Drawing for the job (mm, zero at the part's lowest x, y, z). Give positions to 0.01 mm unless a question says otherwise; leave off trailing zeros. Order: outer loops, then holes, each group sorted by start corner. A loop starts at its lowest first (then second) coordinate and runs counter-clockwise, first axis right, second up. Notation, with made-up numbers: (0, 84.5) - (9, 84.5) arc R18 ccw to (9, 115.5) - close; hole circle Ø10 at (49, 27). An arc over 180 degrees is marked (long way). One line per item, written item: value.
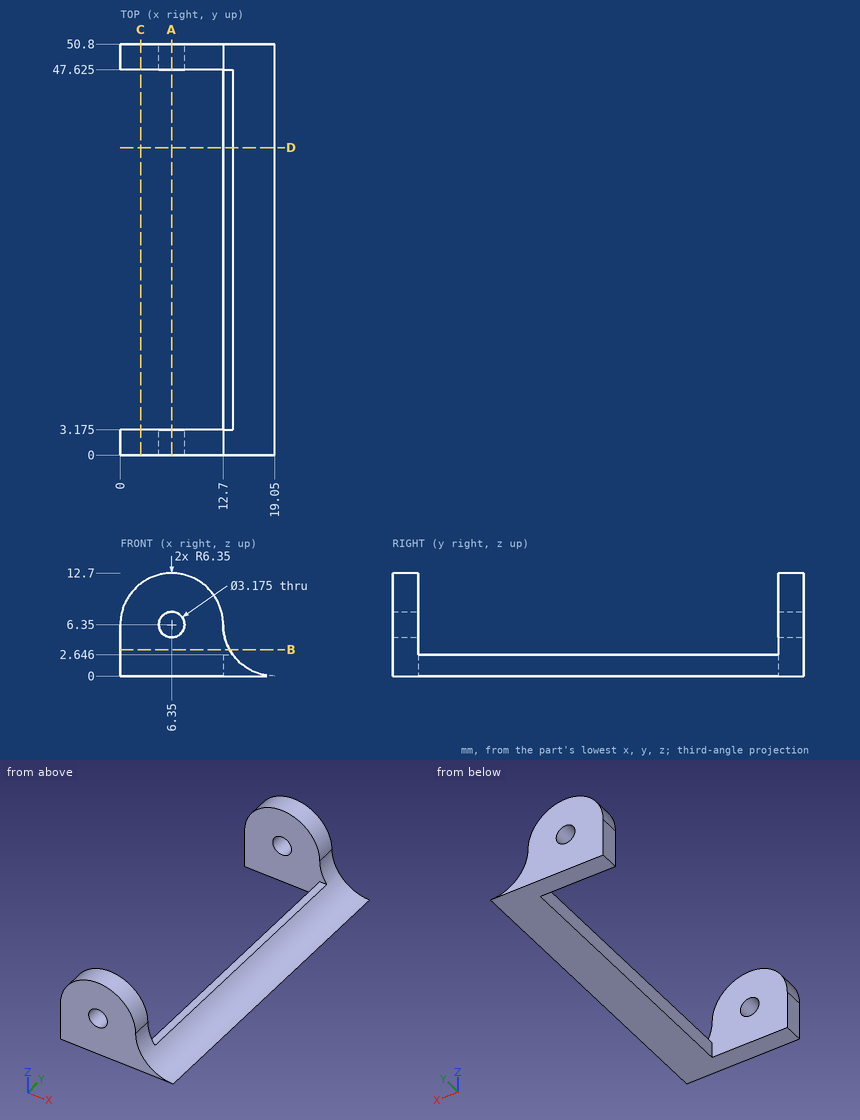
1) Cut at A-A, the plane x = 6.35. Give the cut face in (y, z) (1 decimal).
Outcome:
outline: (0, 0) - (3.2, 0) - (3.2, 4.8) - (0, 4.8) - close; (0, 7.9) - (3.2, 7.9) - (3.2, 12.7) - (0, 12.7) - close; (47.6, 0) - (50.8, 0) - (50.8, 4.8) - (47.6, 4.8) - close; (47.6, 7.9) - (50.8, 7.9) - (50.8, 12.7) - (47.6, 12.7) - close
2) Cut at C-C, the plane x = 2.5. Give the cut face in (y, z) (1 decimal).
Outcome:
outline: (0, 0) - (3.2, 0) - (3.2, 11.4) - (0, 11.4) - close; (47.6, 0) - (50.8, 0) - (50.8, 11.4) - (47.6, 11.4) - close
3) Drill centre lines: line 1 along Z through (x, y) = (6.35, 1.65); line 2 along Y through (x, z) = (10.75, 4.75) (3 decimals); line 3 along X through (y, z) = (48, 6.5). Where is each one in solid material? Low to high. Write a range as from..to.
Outcome:
line 1: z = 0..4.76, 7.94..12.7
line 2: y = 0..3.175, 47.625..50.8
line 3: x = 0..4.77, 7.93..12.7
4) Cut at D-D, the plane y = 38. Give the cut face in (x, z).
Outcome:
outline: (12.7, 0) - (19.05, 0) arc R6.35 cw to (13.89, 2.65) - (12.7, 2.65) - close
5) Pin check, flat tips, straight feed: pin 1 (1.5 mm diameter, centred on x = 10.5, y = 41.5, fed in from -Z); pin 2 (1 mm diameter, centred on x = 13.5, y = 17, fed in from +Z); pin 3 (2 mm diameter, centred on y = 18.5, z = 1.5, fed in from -X). Stop position of each tip, or through.
Outcome:
pin 1: passes through
pin 2: stops at z = 2.65
pin 3: stops at x = 12.7
6) Cut at B-B, the plane z = 3.25. Give the cut face in (x, y) (3 decimals), then the cut area to 3 significant figures.
Outcome:
outline: (0, 0) - (13.508, 0) - (13.508, 3.175) - (0, 3.175) - close; (0, 47.625) - (13.508, 47.625) - (13.508, 50.8) - (0, 50.8) - close
area: 85.8 mm^2
